```python
from build123d import *

# Parameters (mm, degrees)
SKETCH1_R           = 9.625
SKETCH1_W           = 20
SKETCH1_H           = 18
BOSS_EXTRUDE1_DEPTH = 12
SKETCH2_R           = 2.25
CUT_EXTRUDE1_DEPTH  = 104.537432844


with BuildPart() as part:
    # Sketch1 → Boss-Extrude1 (new body)
    with BuildSketch(Plane.XY):
        with BuildLine():
            Line((0, 15), (85, 15))
            ThreePointArc((85, 15), (100, 0), (85, -15))
            Line((85, -15), (0, -15))
            Line((0, -15), (0, -9))
            Line((0, -9), (-10, -9))
            Line((-10, -9), (-14.358898944, 0))
            Line((-14.358898944, 0), (-10, 9))
            Line((-10, 9), (0, 9))
            Line((0, 9), (0, 15))
        make_face()
        with Locations((85, 0)):
            Circle(SKETCH1_R, mode=Mode.SUBTRACT)
        with Locations((22.884427269, 0)):
            Rectangle(SKETCH1_W, SKETCH1_H, mode=Mode.SUBTRACT)
        with Locations((54.884427269, 0)):
            Rectangle(SKETCH1_W, SKETCH1_H, mode=Mode.SUBTRACT)
    extrude(amount=BOSS_EXTRUDE1_DEPTH)

    # Sketch2 → Cut-Extrude1 (cut, through all)
    with BuildSketch(Plane.XZ.offset(9)):
        with Locations((-4, 6)):
            Circle(SKETCH2_R)
    extrude(amount=-CUT_EXTRUDE1_DEPTH, mode=Mode.SUBTRACT)


solid = part.part
```
Source: CAD feature listing. Evaluate the final solid. Frame: model axes, mm. A direction names the side the tool comes from. Coordinates: 2 decimals unless noted, no trailing zeros. Order: outer loops, then holes, each group sorted by start corner. A loop starts at its lowest first (then second) coordinate and runs counter-clockwise, first axis right, second up. Notation, with made-up numbers: (67.5, -19) - (113.5, -19) arc R16 ccw to (113.5, -11) - close; hole circle Ø2 at (12, 56.25). An arc over 180 degrees is marked (long way). One line per item, written item: value.
1) Reachability of faces 1 (the face through (55, -9, 6)), 2 (the face through (0, 12, 6)), 3 (the face through (-6, -9, 4.6)), 4 (the face through (100, 0, 6)) from +Z, -Z, +X, -X, +Y, -Y: full face, straight path, thin tool, end or side. Return the list, or none.
Computed values:
face 1: +Z, -Z
face 2: +Z, -Z, -X, +Y
face 3: +Z, -Z, -X, -Y
face 4: +Z, -Z, +X
2) Cut plane A-A on z = 6. Output: boundary loops of the cut face in (x, y) (3 decimals).
Computed values:
outline: (-14.359, 0) - (-10, -9) - (-6.25, -9) - (-6.25, 9) - (-10, 9) - close; (-1.75, -9) - (0, -9) - (0, -15) - (85, -15) arc R15 ccw to (85, 15) - (0, 15) - (0, 9) - (-1.75, 9) - close; hole (12.884, -9) - (32.884, -9) - (32.884, 9) - (12.884, 9) - close; hole (44.884, -9) - (64.884, -9) - (64.884, 9) - (44.884, 9) - close; hole circle Ø19.25 at (85, 0)
3) Mould query, pull axis Y, two halves, no side actions, for faces 5 (the face through (43, -15, 6)), 6 (the face through (44, 0, 0)), 7 (the face through (32.884, 0, 6)). Classes: released by +Y, released by -Y, zero draft, split by the parting line, or undercut.
Computed values:
face 5: released by -Y
face 6: zero draft
face 7: undercut
4) Cut plane D-D on y = -11. Output: boundary loops of the cut face in (x, z), plus the area to 3 significant figures.
Computed values:
outline: (0, 0) - (95.2, 0) - (95.2, 12) - (0, 12) - close
area: 1,140 mm^2
5) Cut plane B-B on x = 48. Output: boundary loops of the cut face in (y, z), plus the area to 3 significant figures.
Computed values:
outline: (-15, 0) - (-9, 0) - (-9, 12) - (-15, 12) - close; (9, 0) - (15, 0) - (15, 12) - (9, 12) - close
area: 144 mm^2
6) Contact query for flat-ended pins moving along their axis: pin 1 (4 mm diameter, centred on y = -2.5, z = 5, fed in from +X); pin 2 (3 mm diameter, centred on x = -6, z = 7.5, fed in from +Y); pin 3 (5 mm diameter, centred on y = 12, z = 5.5, fed in from -X); pin 4 (2.5 mm diameter, centred on x = -4, z = 6, fed in from -Y). Output: stop coordinate, or through.
Computed values:
pin 1: stops at x = 99.99
pin 2: stops at y = 9
pin 3: stops at x = 0
pin 4: passes through
7) Cut plane C-C on x = 91. Output: boundary loops of the cut face in (y, z), plus the area to 3 significant figures.
Computed values:
outline: (-13.75, 0) - (-7.53, 0) - (-7.53, 12) - (-13.75, 12) - close; (7.53, 0) - (13.75, 0) - (13.75, 12) - (7.53, 12) - close
area: 149 mm^2
8) Ray query, line 1 (Z direction, x = -4, y = 5); line 2 (Y direction, x = 53, z = 0.75); line 3 (X direction, y = -1.5, z = 11.75). Return the intervals inside material, ascending. Write a range as [from, to].
Computed values:
line 1: z = [0, 3.75], [8.25, 12]
line 2: y = [-15, -9], [9, 15]
line 3: x = [-13.63, 12.88], [32.88, 44.88], [64.88, 75.49], [94.51, 99.92]
